Design review of the part built by this model. Coordinates are the model's own, in mm. Give positions to 0.01 mm unless a question says otherwise; leave off trailing zeros. Loops run counter-clockwise (first coordinate to the right, second up) from the corner with the lowest first, then second, coordinate; pieces in that order, holes last.
from build123d import *

# Parameters (mm, degrees)
ESQUISSE1_W             = 100
ESQUISSE1_H             = 100.548113933
ESQUISSE1_R             = 11
BOSS_EXTRU_1_DEPTH      = 5
ESQUISSE2_R             = 1.5
ENL_V_MAT_EXTRU_1_DEPTH = 73.311824759


with BuildPart() as part:
    # Esquisse1 → Boss.-Extru.1 (new body)
    with BuildSketch(Plane.XY):
        with Locations((0, 1.725943033)):
            Rectangle(ESQUISSE1_W, ESQUISSE1_H)
        Circle(ESQUISSE1_R, mode=Mode.SUBTRACT)
    extrude(amount=BOSS_EXTRU_1_DEPTH)

    # Esquisse2 → Enlèv. mat.-Extru.1 (cut, through all)
    with BuildSketch(Plane.XY.offset(5)):
        with BuildLine():
            Line((25, 52), (25, 0))
            ThreePointArc((25, 0), (0, -25), (-25, 0))
            Line((-25, 0), (-25, 52))
            Line((-25, 52), (-50, 52))
            Line((-50, 52), (-50, -48.548113933))
            Line((-50, -48.548113933), (50, -48.548113933))
            Line((50, -48.548113933), (50, 52))
            Line((50, 52), (25, 52))
        make_face()
        with Locations((0, 20)):
            Circle(ESQUISSE2_R)
        with Locations((17.320508076, 10)):
            Circle(ESQUISSE2_R)
        with Locations((17.320508076, -10)):
            Circle(ESQUISSE2_R)
        with Locations((0, -20)):
            Circle(ESQUISSE2_R)
        with Locations((-17.320508076, -10)):
            Circle(ESQUISSE2_R)
        with Locations((-17.320508076, 10)):
            Circle(ESQUISSE2_R)
        with Locations((-12.5, 32)):
            Circle(ESQUISSE2_R)
        with Locations((12.5, 32)):
            Circle(ESQUISSE2_R)
    extrude(amount=-ENL_V_MAT_EXTRU_1_DEPTH, mode=Mode.SUBTRACT)


solid = part.part
Q1. Insertion check: pin 1 (3 mm diameter, centred on x = -9.5, z = 2, fed in from -Y); pin 2 (1 mm diameter, centred on y = -13, z = 2.5, fed in from +X). Each pin has a flat end and moves straight along its axis. Give the tip position at first contact, or say it passes through.
Results:
pin 1: stops at y = -23.69
pin 2: stops at x = 21.65
Q2. Take a section at C-C (y = 20). Give the boundary of the cut face in (x, z), plus the area to 3 significant figures.
Results:
outline: (-25, 0) - (-1.5, 0) - (-1.5, 5) - (-25, 5) - close; (1.5, 0) - (25, 0) - (25, 5) - (1.5, 5) - close
area: 235 mm2
Q3. Draft analysis for pull direction Y (two halves, no side actions). For faces 1 (the face through (0.55, -24.994, 2.535)), 2 (the face through (-15.935, 9.425, 2.535)), 3 (the face through (0, 52, 2)), state which applies: pulls with the +Y half, pulls with the -Y half, needs draft (parallel to the pull), parting line crosses it, or undercut.
Results:
face 1: pulls with the -Y half
face 2: undercut
face 3: pulls with the +Y half
Q4. Wall thickness on line 1 (Y direction, x = 0, z = 2.3); line 2 (Y direction, x = 17, z = 2.7); line 3 (Y direction, x = 16, z = 1.7): over which ranges is each line inside the solid? List them lowest first.
Results:
line 1: y = -25 to -21.5, -18.5 to -11, 11 to 18.5, 21.5 to 52
line 2: y = -18.33 to -11.47, -8.53 to 8.53, 11.47 to 52
line 3: y = -19.21 to -10.71, -9.29 to 9.29, 10.71 to 52
Q5. Take a section at A-A (y = 32). Give the boundary of the cut face in (x, z), plus the area to 3 significant figures.
Results:
outline: (-25, 0) - (-14, 0) - (-14, 5) - (-25, 5) - close; (-11, 0) - (11, 0) - (11, 5) - (-11, 5) - close; (14, 0) - (25, 0) - (25, 5) - (14, 5) - close
area: 220 mm2
Q6. Take a section at B-B (x = 0). Give the boundary of the cut face in (y, z).
Results:
outline: (-25, 0) - (-21.5, 0) - (-21.5, 5) - (-25, 5) - close; (-18.5, 0) - (-11, 0) - (-11, 5) - (-18.5, 5) - close; (11, 0) - (18.5, 0) - (18.5, 5) - (11, 5) - close; (21.5, 0) - (52, 0) - (52, 5) - (21.5, 5) - close
Q7. Take a section at D-D (z = 3.55). Give the number of separate pieces and of enclosed holes in the cut face, plus the area to 3 significant figures.
Results:
separate pieces: 1
enclosed holes: 9
area: 3,150 mm2
